Here's how the part is built. I have some questions about the finished solid (model axes, mm). A direction names the side the tool comes from. Round coordinates to 2 decimals unless told otherwise and drop trailing zeros. Loops run counter-clockwise (first coordinate to the right, second up) from the corner with the lowest first, then second, coordinate; pieces in that order, holes last. Notation, with made-up numbers: (10.5, 32) -> (17.5, 32) arc R7 ccw to (17.5, 38) -> close; hole circle Ø5 at (22.25, -30). An arc over 180 degrees is marked (long way). Use one line per item in the form item = value. Start each with the question number.
Item 1: I'm going to push flat-ended pins straight in: pin 1 Ø1.5 at (x, z) = (32, 3.5) entering from +Y; pin 2 Ø3 at (x, z) = (25.5, -3.5) entering from -Y; pin 3 Ø1.5 at (x, z) = (44, -3) entering from -Y. Where does each tip first touch, or does it pass through?
Item 2: If we section it at A-A (x = 9): Write out the boundary of the cut face in (y, z), then the cut area to 3 significant figures.
Item 3: For faces 5 (the face through (3.6, 0, 0)), 6 (the face through (22.582, -1.802, 5.723)), which set-ups out of +Z, -Z, +X, -X, +Y, -Y let a thin tool reach every point of the face, with its end or its side?
Item 4: If I drill on L1, parallel to Z at x = 42, y = 1; L2, parallel to Z at x = 8, y = -3.25; L3, parallel to Y at x = 39, z = -0.5, over which ranges is the centre line in solid material (lowest first)? Write a range as [from, to].
Item 5: Thinking about a two-plate mould opening in Y: for faces 1 (the face through (48.375, 0.989, -1.289)), 2 (the face through (0.097, 5.202, -0.102)), 3 (the face through (2, 1, 0)), 4 (the face through (2, -1, 0)), which applies, released by +Y, released by -Y, zero draft, split by the parting line, or undercut?
```python
from build123d import *

# Parameters (mm, degrees)
SKETCH2_W  = 12
SKETCH2_H  = 2
SLOT_DEPTH = 3.6


with BuildPart() as part:
    # BodySke → BaseBody (revolve)
    with BuildSketch(Plane.XY, mode=Mode.PRIVATE) as basebody_sk:
        Polygon((0, 0), (0, 5.036), (0.556565659, 6), (44, 6), (50, 0), align=None)
    revolve(basebody_sk.sketch.rotate(Axis((-12.7, 0, 0), (1, 0, 0)), 90), axis=Axis((-12.7, 0, 0), (1, 0, 0)))

    # Sketch2 → Slot (cut)
    with BuildSketch(Plane.ZY):
        Rectangle(SKETCH2_W, SKETCH2_H)
    extrude(amount=-SLOT_DEPTH, mode=Mode.SUBTRACT)


solid = part.part
```
Values found:
q1.pin_1 = 5.33
q1.pin_2 = -5.66
q1.pin_3 = -5.56
q2.outline = circle Ø12 at (0, 0)
q2.area = 113 mm2
q3.face_5 = +Z, -Z, -X
q3.face_6 = +X, -X
q4.L1 = [-5.92, 5.92]
q4.L2 = [-5.04, 5.04]
q4.L3 = [-5.98, 5.98]
q5.face_1 = split by the parting line
q5.face_2 = released by +Y
q5.face_3 = undercut
q5.face_4 = undercut
